Read the model definition and answer for the solid it produces. Units are mm, in the model's axes. A direction names the side the tool comes from. Give positions to 0.01 mm unless a question says otherwise; leave off trailing zeros. Write each loop counter-clockwise with the first axis right and the second up, starting at its lowest first coordinate (ties: lowest second). Pieces come first, ordered by that corner, then holes. Notation, with made-up numbers: M -26,89 L 20,89 A21 cw 20,125 Z; hole C 88.5,72.25 d5. An arc over 180 degrees is marked long. Use a Markdown table: item, result. Add a question column.
Item 1: A cutting plane is placed at A-A on z = 20. Determine the outline of the cut face in (x, y).
Item 2: A cutting plane is placed at B-B on x = -105.5. Determine the outline of the cut face in (y, z), then the cut area to 3 significant figures.
Item 3: For faces 5 (the cylindrical face through (-116.41, 136.32, 37.22)), 6 (the flat face through (-87, 101.326, 39)), 7 (the flat face through (-87, 102.326, 30)), determine the directions among +Z, -Z, +X, -X, +Y, -Y from which every point of the face is accessible in a straight line to the end or side of a thin tool.
Item 4: A cutting plane is placed at D-D on x = -84.5. Determine the outline of the cut face in (y, z), then the cut area to 3 significant figures.
Item 5: Consider probe 1 along X at (y, z) = (176, 20); probe 2 along Y at (x, z) = (-101, 37); probe 3 along Z at (x, y) = (-102, 178.5). Determine where each line is inside the solid, lowest interval first. Write a range as [from, to].
Item 6: A cutting plane is placed at C-C on y = 133.5. Determine the outline of the cut face in (x, z), then the cut area to 3 significant figures.
Item 7: The mould has two halves that part along X. Classify faces 1 (the flat face through (-119.371, 150, 19)), 2 (the flat face through (-86.92, 130.81, 41.13)), 3 (the flat face through (-87, 161, 28)), 4 (the cylindrical face through (-109.96, 197.19, 40.37)): pulls with the +X half, pulls with the -X half, needs draft (parallel to the pull), parting line crosses it, or undercut.
Item 8: Given P1, Ø7, axis at x = -67.37, z = 37, coming from the -Y side; P2, Ø10, axis at x = -107.37, z = 37, coming from the +Y side; P3, Ø6, axis at y = 131.33, z = 37, coming from the -X side; P4, Ø1.5, axis at x = -102.5, y = 171, coming from the +Z side, each flat-ended and moving along its own axis, determine where each tip first touches the part or whether it passes through.
from build123d import *

# Parameters (mm, degrees)
SKETCH4_W              = 64
SKETCH4_H              = 112
BOSS_EXTRUDE1_DEPTH    = 46
CUT_EXTRUDE1_DEPTH     = 18
CUT_EXTRUDE2_DEPTH     = 90
SKETCH7_R              = 5.25
CUT_EXTRUDE3_DEPTH     = 273
M10_TAPPED_HOLE2_D     = 8.5
M10_TAPPED_HOLE2_DEPTH = 50
M10_TAPPED_HOLE2_TIP   = 2.553657631
SKETCH10_R             = 5
CUT_EXTRUDE4_DEPTH     = 6
SKETCH12_R             = 4
CUT_EXTRUDE5_DEPTH     = 50
FILLET1_R              = 2


with BuildPart() as part:
    # Sketch4 → Boss-Extrude1 (new body)
    with BuildSketch(Plane.XY):
        with Locations((-87.370786517, 151.325842697)):
            Rectangle(SKETCH4_W, SKETCH4_H)
    extrude(amount=BOSS_EXTRUDE1_DEPTH)

    # Sketch5 → Cut-Extrude1 (cut)
    with BuildSketch(Plane.XY.offset(46)):
        Polygon((-119.370786517, 187.325842697), (-55.370786517, 187.325842697), (-55.370786517, 119.325842697), (-119.370786517, 142.61993769), align=None)
    extrude(amount=-CUT_EXTRUDE1_DEPTH, mode=Mode.SUBTRACT)

    # Sketch6 → Cut-Extrude2 (cut)
    with BuildSketch(Plane(origin=(-55.370786517, 0, 0), x_dir=(0, 0, -1), z_dir=(1, 0, 0))):
        Polygon((-46, 101.325842697), (-31, 101.325842697), (-31, 102.325842697), (-28, 102.325842697), (-28, 95.325842697), (-46, 95.325842697), align=None)
        Polygon((-12, 95.325842697), (-12, 101.565088044), (-12, 102.325842697), (-9, 102.325842697), (-9, 101.325842697), (0, 101.325842697), (0, 95.325842697), align=None)
    extrude(amount=-CUT_EXTRUDE2_DEPTH, mode=Mode.SUBTRACT)

    # Sketch7 → Cut-Extrude3 (cut)
    with BuildSketch(Plane(origin=(0, 207.325842697, 0), x_dir=(1, 0, 0), z_dir=(0, 1, 0))):
        with Locations(Location((-87.370786517, -20, 0), (0, 0, 270))):
            Circle(SKETCH7_R)
    extrude(amount=-CUT_EXTRUDE3_DEPTH, mode=Mode.SUBTRACT)

    # M10 Tapped Hole2
    with Locations(Plane(origin=(-107.370786517, 207.325842697, 37), x_dir=(0, 0, 1), z_dir=(0, 1, 0))):
        with Locations((0, 0), (0, 40)):
            Hole(M10_TAPPED_HOLE2_D / 2, depth=M10_TAPPED_HOLE2_DEPTH)
            with Locations((0, 0, -(M10_TAPPED_HOLE2_DEPTH + M10_TAPPED_HOLE2_TIP / 2))):  # 118° drill point
                Cone(0, M10_TAPPED_HOLE2_D / 2, M10_TAPPED_HOLE2_TIP, mode=Mode.SUBTRACT)

    # Sketch10 → Cut-Extrude4 (cut)
    with BuildSketch(Plane.ZY.offset(119.370786517)):
        with Locations(Location((37, 131.325842697, 0), (0, 0, 270))):
            Circle(SKETCH10_R)
    extrude(amount=-CUT_EXTRUDE4_DEPTH, mode=Mode.SUBTRACT)

    # Sketch12 → Cut-Extrude5 (cut)
    with BuildSketch(Plane.ZY.offset(113.370786517)):
        with Locations(Location((37, 131.325842697, 0), (0, 0, 270))):
            Circle(SKETCH12_R)
    extrude(amount=-CUT_EXTRUDE5_DEPTH, mode=Mode.SUBTRACT)

    # Fillet1
    fillet1_edges = [part.edges().sort_by_distance(p)[0] for p in [
        (-55.370786517, 110.325842697, 46),
        (-119.370786517, 121.972890193, 46),
        (-119.370786517, 154.325842697, 0),
        (-87.370786517, 207.325842697, 0),
        (-55.370786517, 154.325842697, 0),
        (-55.370786517, 207.325842697, 23),
        (-87.370786517, 207.325842697, 46),
        (-119.370786517, 207.325842697, 23),
    ]]
    fillet(fillet1_edges, radius=FILLET1_R)


solid = part.part
Filled in:
| question | item | result |
|---|---|---|
| 1 | outline | M -119.37,95.33 L -92.62,95.33 L -92.62,207.33 L -117.37,207.33 A2 ccw -119.37,205.33 Z; M -82.12,95.33 L -55.37,95.33 L -55.37,205.33 A2 ccw -57.37,207.33 L -82.12,207.33 Z |
| 2 | outline | M 95.33,12 L 102.33,12 L 102.33,9 L 101.33,9 L 101.33,0 L 205.33,0 A2 ccw 207.33,2 L 207.33,33.18 L 187.33,33.18 L 187.33,28 L 137.57,28 L 137.57,46 L 101.33,46 L 101.33,31 L 102.33,31 L 102.33,28 L 95.33,28 Z; M 187.33,40.82 L 207.33,40.82 L 207.33,44 A2 ccw 205.33,46 L 187.33,46 Z; hole C 131.33,37 d8 |
| 2 | area | 3,870 mm² |
| 3 | face 5 | -X |
| 3 | face 6 | +Z, +X, -X, -Y |
| 3 | face 7 | +X, -X, -Y |
| 4 | outline | M 95.33,12 L 102.33,12 L 102.33,9 L 101.33,9 L 101.33,0 L 205.33,0 A2 ccw 207.33,2 L 207.33,15.6 L 95.33,15.6 Z; M 95.33,24.4 L 207.33,24.4 L 207.33,44 A2 ccw 205.33,46 L 187.33,46 L 187.33,28 L 129.93,28 L 129.93,33.25 A4 cw 129.93,40.75 L 129.93,46 L 101.33,46 L 101.33,31 L 102.33,31 L 102.33,28 L 95.33,28 Z |
| 4 | area | 2,930 mm² |
| 5 | probe 1 | [-119.37, -92.62], [-82.12, -55.37] |
| 5 | probe 2 | [101.33, 127.33], [135.33, 135.93], [187.33, 207.33] |
| 5 | probe 3 | [0, 28] |
| 6 | outline | M -119.37,2 A2 ccw -117.37,0 L -57.37,0 A2 ccw -55.37,2 L -55.37,28 L -94.31,28 L -94.31,33.64 L -113.37,33.64 L -113.37,32.5 L -119.37,32.5 Z; M -119.37,41.5 L -113.37,41.5 L -113.37,40.36 L -94.31,40.36 L -94.31,46 L -117.37,46 A2 ccw -119.37,44 Z; hole C -87.37,20 d10.5 |
| 6 | area | 1,970 mm² |
| 7 | face 1 | pulls with the -X half |
| 7 | face 2 | pulls with the +X half |
| 7 | face 3 | needs draft |
| 7 | face 4 | undercut |
| 8 | P1 | y = 101.33 |
| 8 | P2 | y = 207.33 |
| 8 | P3 | through |
| 8 | P4 | z = 28 |
